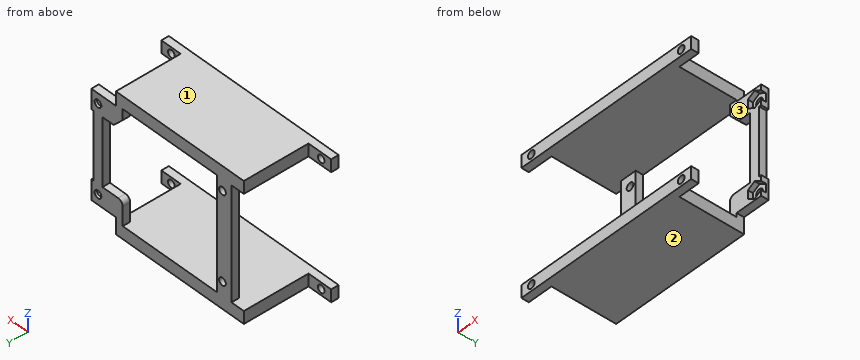
```python
from build123d import *

# Parameters (mm, degrees)
SZKIC1_W                      = 75
SZKIC1_H                      = 5
SZKIC1_R                      = 1.5
DODANIE_WYCI_GNI_CIE1_DEPTH   = 29
DODANIE_WYCI_GNI_CIE1_2_DEPTH = 29
SZKIC2_W                      = 10
SZKIC2_H                      = 5
WYTNIJ_WYCI_GNI_CIE1_DEPTH    = 26
SZKIC3_W                      = 4
SZKIC3_H                      = 55.2
SZKIC3_R                      = 1.5
SZKIC3_W_2                    = 8
DODANIE_WYCI_GNI_CIE6_DEPTH   = 3
SZKIC8_W                      = 2
SZKIC8_H                      = 8
DODANIE_WYCI_GNI_CIE7_DEPTH   = 3
WYTNIJ_WYCI_GNI_CIE3_REACH    = 59.268
SZKIC9_W                      = 4
SZKIC9_H                      = 6.6
SZKIC9_H_2                    = 5.6
WYTNIJ_WYCI_GNI_CIE4_DEPTH    = 2
WYTNIJ_WYCI_GNI_CIE5_START    = -3
SZKIC11_W                     = 1.1
SZKIC11_H                     = 43
WYTNIJ_WYCI_GNI_CIE5_DEPTH    = 3
SZKIC12_W                     = 5
SZKIC12_H                     = 23
DODANIE_WYCI_GNI_CIE8_DEPTH   = 1.5
WYTNIJ_WYCI_GNI_CIE6_REACH    = 58.487
ZAOKR_GLENIE1_R               = 2
WYTNIJ_WYCI_GNI_CIE7_REACH    = 58.487
SZKIC14_W                     = 1.5
SZKIC14_H                     = 45.2


with BuildPart() as part:
    # Szkic1 → Dodanie-wyci_gni_cie1 (new body)
    with BuildSketch(Plane(origin=(0, 0, 0), x_dir=(1, 0, 0), z_dir=(0, 1, 0))):
        with Locations((0, 25.1)):
            Rectangle(SZKIC1_W, SZKIC1_H)
        with Locations(Location((-33.1, 25.1, 0), (0, 0, 90))):
            Circle(SZKIC1_R, mode=Mode.SUBTRACT)
        with Locations(Location((33.1, 25.1, 0), (0, 0, 90))):
            Circle(SZKIC1_R, mode=Mode.SUBTRACT)
    extrude(amount=DODANIE_WYCI_GNI_CIE1_DEPTH)


with BuildPart() as body_2:
    # Szkic1 → Dodanie-wyci_gni_cie1 2 (new body)
    with BuildSketch(Plane(origin=(0, 0, 0), x_dir=(1, 0, 0), z_dir=(0, 1, 0))):
        with Locations((0, -25.1)):
            Rectangle(SZKIC1_W, SZKIC1_H)
        with Locations(Location((33.1, -25.1, 0), (0, 0, 90))):
            Circle(SZKIC1_R, mode=Mode.SUBTRACT)
        with Locations(Location((-33.1, -25.1, 0), (0, 0, 90))):
            Circle(SZKIC1_R, mode=Mode.SUBTRACT)
    extrude(amount=DODANIE_WYCI_GNI_CIE1_2_DEPTH)


with BuildPart() as wytnij_wyci_gni_cie1_tool:
    # Szkic2 → Wytnij-wyci_gni_cie1 (new body)
    with BuildSketch(Plane(origin=(0, 29, 0), x_dir=(1, 0, 0), z_dir=(0, 1, 0))):
        with Locations((-32.5, 25.1)):
            Rectangle(SZKIC2_W, SZKIC2_H)
        with Locations((32.5, 25.1)):
            Rectangle(SZKIC2_W, SZKIC2_H)
        with Locations((32.5, -25.1)):
            Rectangle(SZKIC2_W, SZKIC2_H)
        with Locations((-32.5, -25.1)):
            Rectangle(SZKIC2_W, SZKIC2_H)
    extrude(amount=-WYTNIJ_WYCI_GNI_CIE1_DEPTH)


with BuildPart() as part_1:
    add(part.part)

    # Wytnij-wyci_gni_cie1: cut by wytnij_wyci_gni_cie1_tool
    add(wytnij_wyci_gni_cie1_tool.part, mode=Mode.SUBTRACT)



with BuildPart() as body_2_1:
    add(body_2.part)

    # Wytnij-wyci_gni_cie1: cut by wytnij_wyci_gni_cie1_tool
    add(wytnij_wyci_gni_cie1_tool.part, mode=Mode.SUBTRACT)


with BuildPart() as part_2:
    add(part_1.part)

    add(body_2_1.part)  # Dodanie-wyci_gni_cie6 merges body 2
    # Szkic3 → Dodanie-wyci_gni_cie6 (add)
    # profile 1 of 2: a face of its own
    with BuildSketch(Plane(origin=(0, 29, 0), x_dir=(1, 0, 0), z_dir=(0, 1, 0))):
        with Locations((36.95, 0)):
            Rectangle(SZKIC3_W, SZKIC3_H)
        with Locations(Location((36.95, -18, 0), (0, 0, 270))):
            Circle(SZKIC3_R, mode=Mode.SUBTRACT)
        with Locations(Location((36.95, 17, 0), (0, 0, 270))):
            Circle(SZKIC3_R, mode=Mode.SUBTRACT)
    # profile 2 of 2: a face of its own
    with BuildSketch(Plane(origin=(0, 29, 0), x_dir=(1, 0, 0), z_dir=(0, 1, 0))):
        with Locations((-18.05, 0)):
            Rectangle(SZKIC3_W_2, SZKIC3_H)
        with Locations(Location((-18.05, -18, 0), (0, 0, 270))):
            Circle(SZKIC3_R, mode=Mode.SUBTRACT)
        with Locations(Location((-18.05, 17, 0), (0, 0, 270))):
            Circle(SZKIC3_R, mode=Mode.SUBTRACT)
    extrude(amount=-DODANIE_WYCI_GNI_CIE6_DEPTH)

    # Szkic8 → Dodanie-wyci_gni_cie7 (add)
    with BuildSketch(Plane(origin=(0, 29, 0), x_dir=(1, 0, 0), z_dir=(0, 1, 0))):
        Polygon((29, 21), (29, 27.6), (27.5, 27.6), (27.5, 22.6), (26, 22.6), (26, 13), (34.95, 13), (34.95, 21), align=None)
        with Locations((39.95, 17)):
            Rectangle(SZKIC8_W, SZKIC8_H)
        Polygon((34.95, -22), (34.95, -14), (26, -14), (26, -22.6), (27.5, -22.6), (27.5, -27.6), (29, -27.6), (29, -22), align=None)
        with Locations((39.95, -18)):
            Rectangle(SZKIC8_W, SZKIC8_H)
    extrude(amount=-DODANIE_WYCI_GNI_CIE7_DEPTH)

    # Szkic9 → Wytnij-wyci_gni_cie3 (cut, up to next)
    with BuildSketch(Plane(origin=(0, 29, 0), x_dir=(1, 0, 0), z_dir=(0, 1, 0)), mode=Mode.PRIVATE) as wytnij_wyci_gni_cie3_sk1:
        with Locations((36.95, 24.3)):
            Rectangle(SZKIC9_W, SZKIC9_H)
    wytnij_wyci_gni_cie3_tool1 = extrude(wytnij_wyci_gni_cie3_sk1.sketch, amount=-WYTNIJ_WYCI_GNI_CIE3_REACH, mode=Mode.PRIVATE) & part_2.part
    # Szkic9 → Wytnij-wyci_gni_cie3 (cut, up to next)
    with BuildSketch(Plane(origin=(0, 29, 0), x_dir=(1, 0, 0), z_dir=(0, 1, 0)), mode=Mode.PRIVATE) as wytnij_wyci_gni_cie3_sk2:
        with Locations((36.95, -24.8)):
            Rectangle(SZKIC9_W, SZKIC9_H_2)
    wytnij_wyci_gni_cie3_tool2 = extrude(wytnij_wyci_gni_cie3_sk2.sketch, amount=-WYTNIJ_WYCI_GNI_CIE3_REACH, mode=Mode.PRIVATE) & part_2.part
    add(wytnij_wyci_gni_cie3_tool1.solids().sort_by_distance((36.95, 29, -24.3))[0], mode=Mode.SUBTRACT)
    add(wytnij_wyci_gni_cie3_tool2.solids().sort_by_distance((36.95, 29, 24.8))[0], mode=Mode.SUBTRACT)

    # Szkic10 → Wytnij-wyci_gni_cie4 (cut)
    with BuildSketch(Plane.XZ.offset(-26)):
        Polygon((36.95, -13.593633412), (34, -15.296816706), (34, -18.703183294), (36.95, -20.406366588), (39.9, -18.703183294), (39.9, -15.296816706), align=None)
        Polygon((36.95, 21.406366588), (34, 19.703183294), (34, 16.296816706), (36.95, 14.593633412), (39.9, 16.296816706), (39.9, 19.703183294), align=None)
    extrude(amount=-WYTNIJ_WYCI_GNI_CIE4_DEPTH, mode=Mode.SUBTRACT)

    # Szkic11 → Wytnij-wyci_gni_cie5 (cut)
    with BuildSketch(Plane(origin=(0, 29, 0), x_dir=(1, 0, 0), z_dir=(0, 1, 0)).offset(WYTNIJ_WYCI_GNI_CIE5_START)):
        with Locations((40.4, -0.5)):
            Rectangle(SZKIC11_W, SZKIC11_H)
    extrude(amount=WYTNIJ_WYCI_GNI_CIE5_DEPTH, mode=Mode.SUBTRACT)

    # Szkic12 → Dodanie-wyci_gni_cie8 (add)
    with BuildSketch(Plane(origin=(27.5, 0, 0), x_dir=(0, 0, -1), z_dir=(1, 0, 0))):
        with Locations((-25.1, 14.5)):
            Rectangle(SZKIC12_W, SZKIC12_H)
        with Locations((25.1, 14.5)):
            Rectangle(SZKIC12_W, SZKIC12_H)
    extrude(amount=DODANIE_WYCI_GNI_CIE8_DEPTH)

    # Szkic13 → Wytnij-wyci_gni_cie6 (cut, up to next)
    with BuildSketch(Plane(origin=(0, 29, 0), x_dir=(1, 0, 0), z_dir=(0, 1, 0)), mode=Mode.PRIVATE) as wytnij_wyci_gni_cie6_sk1:
        Polygon((26, -14), (30, -14), (26, -18.3), align=None)
    wytnij_wyci_gni_cie6_tool1 = extrude(wytnij_wyci_gni_cie6_sk1.sketch, amount=-WYTNIJ_WYCI_GNI_CIE6_REACH, mode=Mode.PRIVATE) & part_2.part
    add(wytnij_wyci_gni_cie6_tool1.solids().sort_by_distance((27.333333, 29, 15.433333))[0], mode=Mode.SUBTRACT)

    # Zaokr_glenie1
    zaokr_glenie1_edges = [part_2.edges().sort_by_distance(p)[0] for p in [
        (26, 27.5, -13),
    ]]
    fillet(zaokr_glenie1_edges, radius=ZAOKR_GLENIE1_R)

    # Szkic14 → Wytnij-wyci_gni_cie7 (cut, up to next)
    with BuildSketch(Plane(origin=(0, 29, 0), x_dir=(1, 0, 0), z_dir=(0, 1, 0)), mode=Mode.PRIVATE) as wytnij_wyci_gni_cie7_sk1:
        with Locations((-14.8, 0)):
            Rectangle(SZKIC14_W, SZKIC14_H)
    wytnij_wyci_gni_cie7_tool1 = extrude(wytnij_wyci_gni_cie7_sk1.sketch, amount=-WYTNIJ_WYCI_GNI_CIE7_REACH, mode=Mode.PRIVATE) & part_2.part
    add(wytnij_wyci_gni_cie7_tool1.solids().sort_by_distance((-14.8, 29, 0))[0], mode=Mode.SUBTRACT)


solid = part_2.part
```
The listing builds one solid part. Answer for the finished solid, in the listing's coordinates (mm). Face numbers are marked on the shaded views. Coordinates: 2 decimals unless noted, no trailing zeros. Loops run counter-clockwise (first coordinate to the right, second up) from the corner with the lowest first, then second, coordinate; pieces in that order, holes last. Notation, with made-up numbers: M -37.75,-14.5 L -26.75,-14.5 A30 cw -26.75,22.5 Z; hole C 88,54.5 d5. An arc over 180 degrees is marked long. Answer as CSV lines item,"result". Start each with the question number.
(1) The mould has two halves that part along Z. Classify the marked faces 1, 2 and 3: pulls with the +Z half, pulls with the -Z half, needs draft (parallel to the pull), parting line crosses it, or undercut.
(2) The part is cut by section A-A (z = 5.5). Give the vertices of the cut face in (x, y).
(3) The part is cut by section C-C (x = -18.05). Give the vertices of the cut face in (y, z).
(4) Given pin 1 (1.5 mm diameter, centred on x = 32.5, y = 27.5, fed in from +Z); pin 2 (0.7 mm diameter, centred on x = 39.5, y = 27.5, fed in from -Z); pin 3 (1.5 mm diameter, centred on y = 27, z = -4, fed in from -X), each flat-ended and moving along its own axis, determine where each tip first touches the part or whether it passes through.
(5) The part is cut by section D-D (y = 19.5). Give the vertices of the cut face in (x, z).
(6) Find the intervals of material crossed by L1, parallel to Z at x = 33.1, y = 2.1; L2, parallel to X at y = 2, z = -25.1; L3, parallel to X at y = 28.4, z = -17, in increasing order. Write a range as [from, to].
(7) The part is cut by section B-B (z = -17). Give the vertices of the cut face in (x, y).
Determined:
1,face 1,"pulls with the +Z half"
1,face 2,"pulls with the -Z half"
1,face 3,"undercut"
2,outline,"M -22.05,26 L -15.55,26 L -15.55,29 L -22.05,29 Z; M 34.95,26 L 38.95,26 L 38.95,29 L 34.95,29 Z"
3,outline,"M 0,-27.6 L 29,-27.6 L 29,-18.5 L 26,-18.5 L 26,-22.6 L 0,-22.6 Z; M 0,22.6 L 26,22.6 L 26,19.5 L 29,19.5 L 29,27.6 L 0,27.6 Z; M 26,-15.5 L 29,-15.5 L 29,16.5 L 26,16.5 Z"
4,pin 1,"z = 22"
4,pin 2,"z = -21"
4,pin 3,"x = -22.05"
5,outline,"M -27.5,-27.6 L 29,-27.6 L 29,-22.6 L -27.5,-22.6 Z; M -27.5,22.6 L 29,22.6 L 29,27.6 L -27.5,27.6 Z"
6,L1,"[-27.6, -26.6], [-23.6, -22.6], [22.6, 23.6], [26.6, 27.6]"
6,L2,"[-37.5, -34.6], [-31.6, 31.6], [34.6, 37.5]"
6,L3,"[-22.05, -19.55], [-16.55, -15.55], [26, 35.45], [38.45, 39.85]"
7,outline,"M -22.05,26 L -19.55,26 L -19.55,29 L -22.05,29 Z; M -16.55,26 L -15.55,26 L -15.55,29 L -16.55,29 Z; M 26,26 L 34,26 L 34,28 L 35.45,28 L 35.45,29 L 26,29 Z; M 38.45,28 L 39.85,28 L 39.85,29 L 38.45,29 Z"
